Verification items for the finished model (mm, model axes). A direction names the side the tool comes from. Round coordinates to 2 decimals unless told otherwise and drop trailing zeros. Write each loop counter-clockwise with the first axis right and the second up, starting at its lowest first coordinate (ties: lowest second). Pieces come first, ordered by that corner, then holes. Notation, with made-up numbers: M 38,-18.75 L 80,-18.75 A28 ccw 80,17.25 Z; hole C 56,16.5 d9. An arc over 180 degrees is marked long. One line per question, with ' | ' between items.
Autodesk Inventor part; units mm, degrees
ref_plane "Arbeitsebene1" through (0, 0, 0) normal (0, 0, 1) x (1, 0, 0)
ref_plane "YZ Plane" through (0, 0, 0) normal (1, 0, 0) x (0, 1, 0)
ref_plane "XZ Plane" through (0, 0, 0) normal (0, 1, 0) x (-1, 0, 0)
sketch "Skizze1" plane through (0, 0, 0) normal (0, 0, 1) x (1, 0, 0)
  circle A0 centre (0, 0) radius 21
  circle A1 centre (0, 0) radius 25 construction
  circle A2 centre (-25, 0) radius 1.75
  circle A3 centre (25, 0) radius 1.75
  arc A4 (-27.5875, 2.7143) -> (-27.5875, -2.7143) centre (-25, 0) ccw
  arc A5 (27.5875, -2.7143) -> (27.5875, 2.7143) centre (25, 0) ccw
  line L0 (-27.5875, 2.7143) -> (-14.49, 15.2)
  line L1 (-27.5875, -2.7143) -> (-14.49, -15.2)
  line L2 (14.49, -15.2) -> (27.5875, -2.7143)
  line L3 (14.49, 15.2) -> (27.5875, 2.7143)
  line L4 (-25, 0) -> (25, 0) construction
  circle A6 centre (0, 0) radius 1.5
  dimension "d0" = 42
  dimension "d1" = 3.5
  dimension "d2" = 50
  dimension "d3" = 2
  dimension "d8" = 3
extrude "Extrusion1" add sketch "Skizze1" against normal blind 1.5 contours A0 | A0 L3 A5 L2 | A0 L1 A4 L0 | A6
extrude "Extrusion2" add sketch "Skizze1" against normal blind 20 contours A0 | A6
extrude "Extrusion3" add sketch "Skizze1" along normal blind 10 contours A6
sketch "Skizze2" plane through (0, 0, 0) normal (0, 0, 1) x (1, 0, 0)
  circle A0 centre (0, 0) radius 5
  dimension "d11" = 10
extrude "Extrusion4" add sketch "Skizze2" along normal blind 1
ref_plane "Arbeitsebene1" through (0, 0, 0) normal (0, 0, 1) x (1, 0, 0)
fillet "Rundung1" radius 1 1 edges at (14.49, 15.2, -20)
sketch "Skizze3" plane through (0, 0, -20) normal (0, 0, -1) x (-1, 0, 0)
  circle A0 centre (0, 0) radius 21
  line L0 (-18.963, -9.0226) -> (-8.1058, -19.3726)
  line L1 (-8.1058, -19.3726) -> (-15.0058, -26.6106)
  line L2 (-15.0058, -26.6106) -> (-25.863, -16.2606)
  line L3 (-25.863, -16.2606) -> (-18.963, -9.0226)
  line L4 (0, 0) -> (-20.4344, -21.4356) construction
  circle A1 centre (0, 0) radius 21 construction
  arc A2 (-14.49, 15.2) -> (-14.49, -15.2) centre (0, 0) ccw construction
  line L5 (-14.49, 15.2) -> (-27.5875, 2.7143) construction
  arc A3 (-27.5875, 2.7143) -> (-27.5875, -2.7143) centre (-25, 0) ccw construction
  line L6 (-27.5875, -2.7143) -> (-14.49, -15.2) construction
  circle A4 centre (-25, 0) radius 1.75 construction
  point P0 (-13.5344, -14.1976)
  dimension "d15" = 15
  dimension "d16" = 10
properties part number "Stepper_42mm" material "Aluminium 6061"
1. Mould release check, pull along Y, two halves, no side actions. Record for faces 4 (the face through (23, -1, -1.5)), 5 (the face through (-1.08, 4.88, 0.49)), 6 (the face through (-26.75, 0.08, -0.74)): pulls with the +Y half, pulls with the -Y half, needs draft (parallel to the pull), parting line crosses it, or undercut.
Results:
face 4: needs draft | face 5: parting line crosses it | face 6: undercut
2. Section check C-C, the plane z = -2.5. Record the cut outline in (x, y), then the cut area to 3 significant figures.
Results:
outline: C 0,0 d42 | area: 1,390 mm2
3. Section check A-A, the plane y = 0. Record the cut outline in (x, z).
Results:
outline: M -28.75,-1.5 L -26.75,-1.5 L -26.75,0 L -28.75,0 Z; M -23.25,-1.5 L -21,-1.5 L -21,-19 A1 ccw -20,-20 L 20,-20 A1 ccw 21,-19 L 21,-1.5 L 23.25,-1.5 L 23.25,0 L 5,0 L 5,1 L 1.5,1 L 1.5,10 L -1.5,10 L -1.5,1 L -5,1 L -5,0 L -23.25,0 Z; M 26.75,-1.5 L 28.75,-1.5 L 28.75,0 L 26.75,0 Z
4. Section check D-D, the plane x = 0. Record the cut outline in (y, z).
Results:
outline: M -21,-19 A1 ccw -20,-20 L 20,-20 A1 ccw 21,-19 L 21,0 L 5,0 L 5,1 L 1.5,1 L 1.5,10 L -1.5,10 L -1.5,1 L -5,1 L -5,0 L -21,0 Z
5. Go/stop test with flat-tipped pins: P1, Ø4, axis at x = -25, y = 0, coming from the -Z side; P2, Ø11, axis at x = 1, y = -2, coming from the +Z side; P3, Ø2, axis at y = -3, z = -16, coming from the +X side; P4, Ø6, axis at y = -4, z = -16, coming from the -X side. Record where each tip stops, or that it passes through.
Results:
P1: stops at z = -1.5 | P2: stops at z = 10 | P3: stops at x = 20.9 | P4: stops at x = -20.98
6. Thickness scan on line 1 (Z direction, x = -23.5, y = 2); line 2 (Z direction, x = 0, y = -17); line 3 (Y direction, x = -25, z = -0.7). Record the ranges inside material, lowest first.
Results:
line 1: z = -1.5 to 0 | line 2: z = -20 to 0 | line 3: y = -5.18 to -1.75, 1.75 to 5.18
7. Tool access check on faces 1 (the face through (20.03, 6.31, -9.37)), 2 (the face through (-1.2, 1.2, 1)), 3 (the face through (-21.1, -8.9, -0.7)). Record the directions out of +Z, -Z, +X, -X, +Y, -Y that give a thin tool (end or side, any length) a straight path to the whole face; none if there is none.
Results:
face 1: -Z | face 2: +Z | face 3: +Z, -Z, -X, -Y
8. Section check B-B, the plane x = 25. Record the cut outline in (y, z).
Results:
outline: M -5.18,-1.5 L -1.75,-1.5 L -1.75,0 L -5.18,0 Z; M 1.75,-1.5 L 5.18,-1.5 L 5.18,0 L 1.75,0 Z
